For this review, use the dimensioned drawing (mm, ordinates from the lowest corner) and the shaded views. Round coordinates to 2 decimals unless told otherwise and drop trailing zeros. Loops run counter-clockwise (first coordinate to the right, second up) from the corner with the lowest first, then second, coordinate; pieces in that order, holes last. Notation, with made-up numbers: M 74,-4.75 L 83,-4.75 A13 cw 83,14.25 Z; hole C -14.75,8 d11. An arc over 180 degrees is marked long. Answer as a JSON object with one key per item and string values. Group by question number.
Item 1: The part is to be moulded in two halves that separate along Z. For the marked faces 1, 2 and 3, say which applies: +Z half, -Z half, draft (parallel to the pull), parting line (faces both ways), or undercut.
Item 2: To check wall thickness, follow line 1 (X direction, y = 7.8, z = 0.6); line 2 (Y direction, x = 5.75, z = 1.1); line 3 (Y direction, x = 12, z = 0.3). State the ranges of each line that lie inside material, in increasing order.
Item 3: Consider section A-A (y = 7.8). Give the boundary of the cut face in (x, z), and give its area (3 significant figures).
Item 4: Consider section C-C (z = 0.9). Give the boundary of the cut face in (x, y), and give its area (3 significant figures).
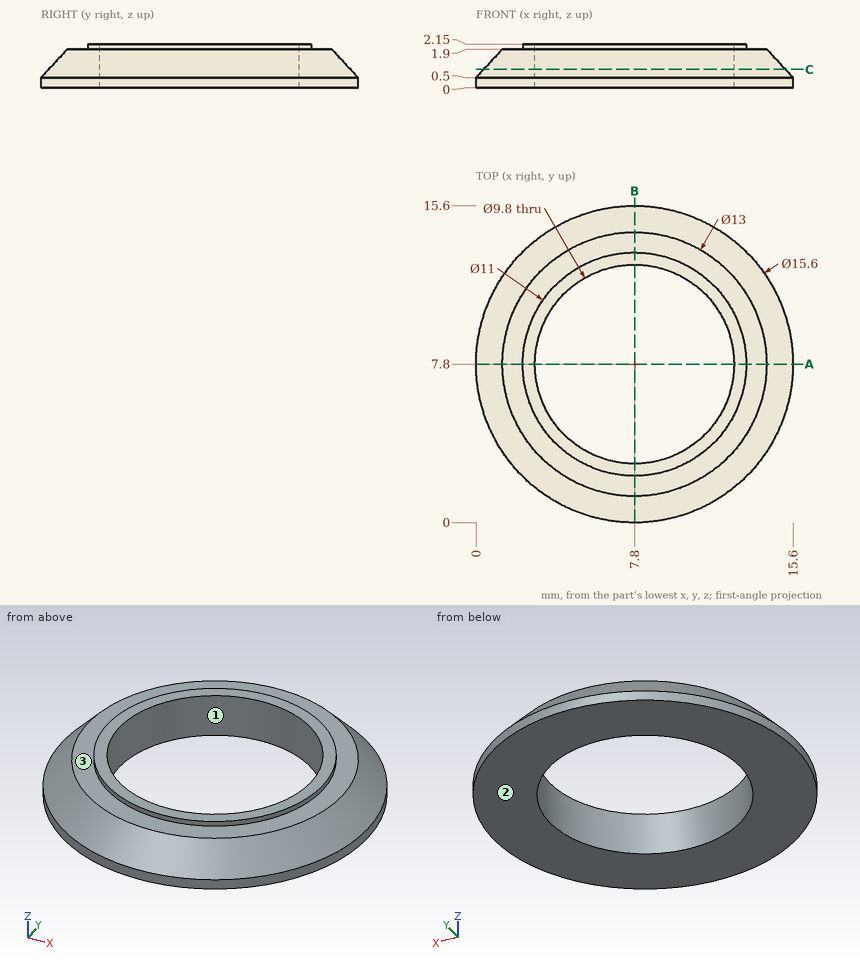
Geometry results:
{
 "1": {"face 1": "draft", "face 2": "-Z half", "face 3": "+Z half"},
 "2": {"line 1": "x = 0.09 to 2.9, 12.7 to 15.51", "line 2": "y = 0.85 to 3.35, 12.25 to 14.75", "line 3": "y = 1.23 to 5.28, 10.32 to 14.37"},
 "3": {"outline": "M 0,0 L 2.9,0 L 2.9,2.15 L 2.3,2.15 L 2.3,1.9 L 1.3,1.9 L 0,0.5 Z; M 12.7,0 L 15.6,0 L 15.6,0.5 L 14.3,1.9 L 13.3,1.9 L 13.3,2.15 L 12.7,2.15 Z", "area": "9.50 mm^2"},
 "4": {"outline": "C 7.8,7.8 d14.86; hole C 7.8,7.8 d9.8", "area": "97.9 mm^2"}
}
